CAD build for the part. Positions are in the model's coordinates, mm. A direction names the side the tool comes from. Round coordinates to 2 decimals unless told otherwise and drop trailing zeros. Write each loop counter-clockwise with the first axis right and the second up, starting at its lowest first coordinate (ties: lowest second). Pieces come first, ordered by that corner, then holes. Notation, with made-up numbers: (-13.75, 29.5) - (-8.75, 29.5) arc R23 ccw to (-8.75, 56.5) - close; hole circle Ø4 at (49, 37.5). An arc over 180 degrees is marked (long way). Answer in a Markdown table with one row per item.
Autodesk Fusion 360 part; units mm, degrees
sketch "Sketch1" plane through (0, 0, 0) normal (0, 0, 1) x (1, 0, 0)
  line L0 (10, 1.5) -> (-10, 1.5)
  line L1 (-10, 1.5) -> (-10, -1.5)
  line L2 (-10, -1.5) -> (10, -1.5)
  line L3 (10, -1.5) -> (10, 1.5)
  dimension "d1" = 20
  dimension "d2" = 3
extrude "Extrude1" add sketch "Sketch1" along normal blind 19
sketch "Sketch2" plane through (0, 1.5, 0) normal (0, 1, 0) x (-1, 0, 0)
  line L0 (-10, 0) -> (10, 0)
  line L1 (10, 0) -> (10, 19)
  line L2 (10, 19) -> (-10, 19)
  line L3 (-10, 19) -> (-10, 0)
  line L4 (0, 9.05) -> (0, 9.05)
  line L5 (-2, 7.05) -> (-2, 0)
  line L6 (2, 7.05) -> (2, 0)
  arc A0 (0, 9.05) -> (-2, 7.05) centre (0, 7.05) ccw
  arc A1 (2, 7.05) -> (0, 9.05) centre (0, 7.05) ccw
  point P0 (0, 9.05)
  dimension "d9" = 2
extrude "Extrude2" cut sketch "Sketch2" against normal blind 3 contours L0 L5 L6 A0 A1
fillet "Fillet1" radius 4 2 edges at (10, 0, 19) (-10, 0, 19)
sketch "Sketch3" plane through (0, 1.5, 0) normal (0, 1, 0) x (-1, 0, 0)
  arc A0 (10, 15) -> (6, 19) centre (6, 15) ccw
  line L0 (6, 19) -> (-6, 19)
  arc A1 (-6, 19) -> (-10, 15) centre (-6, 15) ccw
  line L1 (-10, 15) -> (-10, 0)
  line L2 (-10, 0) -> (-2, 0)
  line L3 (-2, 0) -> (-2, 7.05)
  arc A2 (2, 7.05) -> (-2, 7.05) centre (0, 7.05) ccw
  line L4 (2, 7.05) -> (2, 0)
  line L5 (2, 0) -> (10, 0)
  line L6 (10, 0) -> (10, 15)
  line L7 (0, 19) -> (0, 13.1)
  line L8 (0, 19) -> (0, 17.5)
  line L9 (0, 13.1) -> (0, 14.6)
  ellipse E0 centre (0, 16.05) end of major axis (0, 17.5) minor radius 6.5
  line L10 (0, 14.6) -> (0, 17.5)
  line L11 (6.5, 16.05) -> (-6.5, 16.05)
  dimension "d14" = 5.9
  dimension "d15" = 1.5
  dimension "d16" = 1.5
  dimension "d17" = 13
extrude "Extrude3" cut sketch "Sketch3" against normal blind 3 contours L7 E0 L10 L11 | L7 E0 L10 L11 | L7 E0 L10 L11 | L7 E0 L10 L11
Q1. 3-axis set-ups, long thin cutter, end or side, ignore diameter. For faces 4 (the flat face through (0.1, 1.5, 9.4)), 5 (the flat face through (-2, 0, 4)): which of +Z, -Z, +X, -X, +Y, -Y reach the whole face in a straight line?
Computed:
| item | result |
|---|---|
| face 4 | +Z, -Z, +X, -X, +Y |
| face 5 | -Z, +Y, -Y |
Q2. Saw through at A-A on z = 5.5. List the corners of the cut face in (x, y).
Computed:
| item | result |
|---|---|
| outline | (-10, -1.5) - (-2, -1.5) - (-2, 1.5) - (-10, 1.5) - close; (2, -1.5) - (10, -1.5) - (10, 1.5) - (2, 1.5) - close |
Q3. Pull direction X, two halves, no side cores. Call faces 1 (the cylindrical face through (-0.04, 0.02, 9.05)), 2 (the flat face through (10, 0, 7)), 3 (the flat face through (-0.1, -1.5, 9.4)): released by +X, released by -X, zero draft, split by the parting line, or undercut.
Computed:
| item | result |
|---|---|
| face 1 | undercut |
| face 2 | released by +X |
| face 3 | zero draft |
Q4. Drill centre lines: line 1 (X direction, y = -0.1, z = 6.5); line 2 (Z direction, x = 6.25, y = -0.55); line 3 (Z direction, x = 5.75, y = -0.8). Where is each one in solid material? Low to high.
Computed:
| item | result |
|---|---|
| line 1 | x = -10 to -2, 2 to 10 |
| line 2 | z = 0 to 15.65, 16.45 to 18.99 |
| line 3 | z = 0 to 15.37, 16.73 to 19 |
